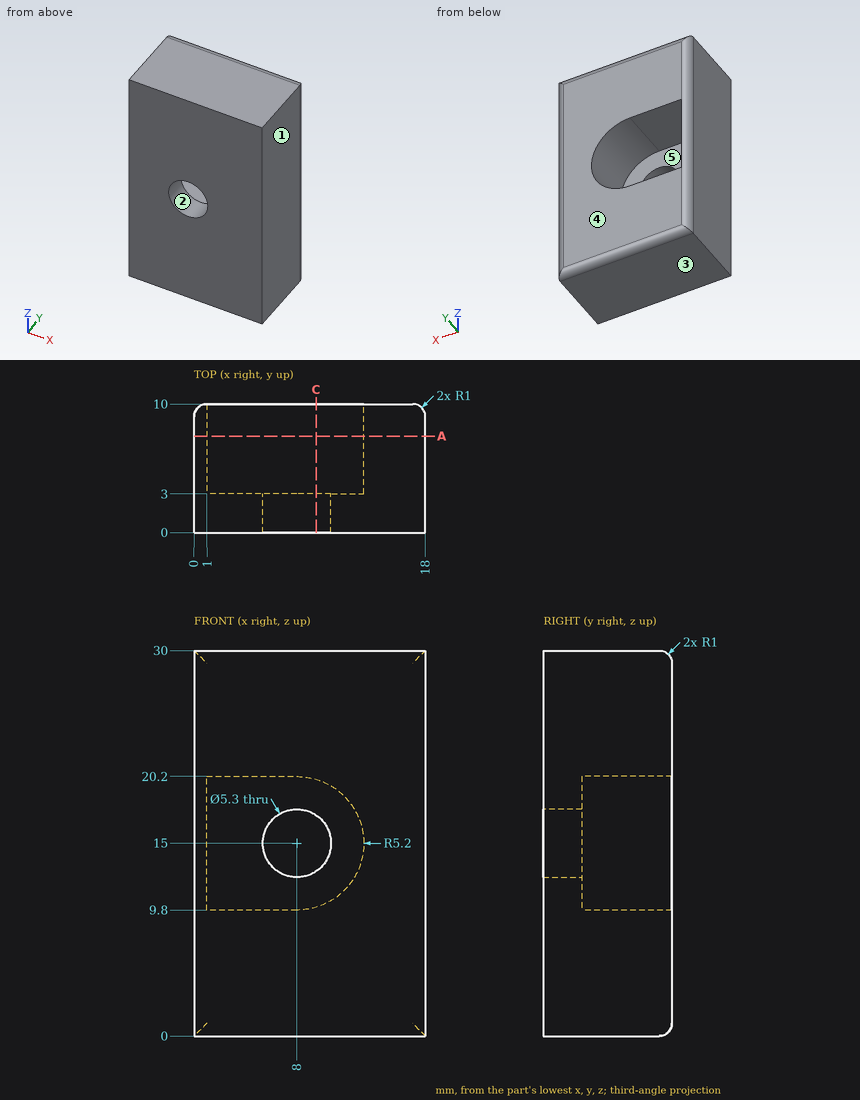
Job drawing, mm, ordinate dimensions from the low corner. One solid piece. A direction names the side the tool comes from. Give positions to 0.01 mm unless a question says otherwise; leave off trailing zeros. Write each loop counter-clockwise with the first axis right and the second up, starting at its lowest first coordinate (ties: lowest second). Pieces come first, ordered by that corner, then holes. Notation, with made-up numbers: M 50.5,3.25 L 109.5,3.25 A16 ccw 109.5,32.25 Z; hole C -4,-38.75 d2. An arc over 180 degrees is marked long. Put each result on its own line as item: value. Start each with the question number.
(1) Flat gauge pin, fed straight in: pin 1 Ø5 at (x, z) = (9.5, 14.5) entering from +Y. Where does the tip first touch, or does it go through?
(2) Mould opens along X. For the marked faces 1, 2 and 3 say: +X half, -X half, draft (parallel to the pull), parting line (faces both ways), or undercut.
(3) Band-saw the part on C-C, the plane x = 9.5. Write the cut outline in (y, z), and give its area (3 significant figures).
(4) Band-saw the part on A-A, the plane y = 7.5. Write the cut outline in (x, z), and give its area (3 significant figures).
(5) Which spindle directions (+Z, -Z, +X, -X, +Y, -Y) get a long thin tool onto all of the face, cutting with end or side? Do the marked faces 4 and 5. Say none if no direction does.
(6) Probe L1, parallel to X at y = 0.8, z = 15; L2, parallel to Z at x = 1.5, y = 9; L3, parallel to X at y = 5.5, z = 13.25. List the from-to ranges inside material, lowest first.
Response values:
1. pin 1: stops at y = 3
2. face 1: +X half
2. face 2: undercut
2. face 3: draft
3. outline: M 0,0 L 9,0 A1 ccw 10,1 L 10,10.02 L 3,10.02 L 3,12.82 L 0,12.82 Z; M 0,17.18 L 3,17.18 L 3,19.98 L 10,19.98 L 10,29 A1 ccw 9,30 L 0,30 Z
3. area: 217 mm2
4. outline: M 0,0 L 18,0 L 18,30 L 0,30 Z; hole M 1,9.8 L 8,9.8 A5.2 ccw 8,20.2 L 1,20.2 Z
4. area: 425 mm2
5. face 4: +Z, -Z, +X, -X, +Y
5. face 5: +Y
6. L1: x = 0 to 5.35, 10.65 to 18
6. L2: z = 0 to 9.8, 20.2 to 30
6. L3: x = 0 to 1, 12.9 to 18
